from build123d import *

# Parameters (mm, degrees)
EXTRUDE_1_DEPTH     = 30
FILLET_1_R          = 1
SKETCH_3_R          = 1.6
CUT_EXTRUDE_1_DEPTH = 4


with BuildPart() as part:
    # 草图1 → 凸台-拉伸1 (new body)
    with BuildSketch(Plane.XY):
        Polygon((-34.18476969, 24.74285776), (-14.18476969, 24.74285776), (-14.18476969, 16.74285776), (-21.48476969, 16.74285776), (-19.68476969, 18.99285776), (-28.68476969, 18.99285776), (-26.88476969, 16.74285776), (-34.18476969, 16.74285776), align=None)
    extrude(amount=EXTRUDE_1_DEPTH)

    # 圆角1
    fillet_1_edges = [part.edges().sort_by_distance(p)[0] for p in [
        (-34.18476969, 24.74285776, 15),
        (-14.18476969, 24.74285776, 15),
        (-14.18476969, 16.74285776, 15),
        (-34.18476969, 16.74285776, 15),
    ]]
    fillet(fillet_1_edges, radius=FILLET_1_R)

    # 草图3 → 切除-拉伸1 (cut)
    with BuildSketch(Plane(origin=(0, 24.74285776, 0), x_dir=(1, 0, 0), z_dir=(0, 1, 0))):
        with Locations(Location((-31.68476969, -10, 0), (0, 0, 270))):
            Circle(SKETCH_3_R)
        with Locations(Location((-31.68476969, -20, 0), (0, 0, 270))):
            Circle(SKETCH_3_R)
        with Locations(Location((-16.68476969, -10, 0), (0, 0, 270))):
            Circle(SKETCH_3_R)
        with Locations(Location((-16.68476969, -20, 0), (0, 0, 270))):
            Circle(SKETCH_3_R)
        with Locations(Location((-24.18476969, -26, 0), (0, 0, 270))):
            Circle(SKETCH_3_R)
    extrude(amount=-CUT_EXTRUDE_1_DEPTH, mode=Mode.SUBTRACT)


solid = part.part
Work out the finished part from the listing and answer in its coordinate system (mm). A direction names the side the tool comes from. Round coordinates to 2 decimals unless told otherwise and drop trailing zeros. Write each loop counter-clockwise with the first axis right and the second up, starting at its lowest first coordinate (ties: lowest second). Pieces come first, ordered by that corner, then holes. Notation, with made-up numbers: (89, 4) -> (135, 4) arc R19 ccw to (135, 35) -> close; hole circle Ø1 at (61, 10). An arc over 180 degrees is marked (long way). Answer as CSV lines item,"result". Start each with the question number.
(1) The part is cut by section C-C, the plane z = 5. Give the vertices of the cut face in (x, y), then the cut area to 3 significant figures.
(2) The part is cut by section B-B, the plane x = -23. Give the vertices of the cut face in (y, z), then the cut area to 3 significant figures.
(3) Find the intervals of material crossed by probe 1 along Z at (x, y) = (-15.25, 21.5); probe 2 along Y at (x, z) = (-24.25, 6.5); probe 3 along Z at (x, y) = (-25.25, 23.25), in increasing order.
(4) A tool of negligible diameter and unlimited length cuts with its end or side. For faces 4 (the flat face through (-27.797, 17.884, 14.79)), 5 (the flat face through (-18, 16.743, 15)), 6 (the flat face through (-17, 20.743, 20)), from which of +Z, -Z, +X, -X, +Y, -Y can it reach the whole face along a straight path? Write none if from no direction.
(5) The mould has two halves that part along X. Classify faces 1 (the flat face through (-24, 18.993, 15)), 2 (the flat face through (-30, 16.743, 15)), 3 (the flat face through (-14.185, 21, 15)): +X half, -X half, draft (parallel to the pull), parting line (faces both ways), or undercut.
(6) The part is cut by section D-D, the plane z = 20. Give the vertices of the cut face in (x, y).
(7) Each of these flat-tipped pins is pushed along its axis until it touches: pin 1 (2.5 mm diameter, centred on x = -26.5, z = 11.5, fed in from -Y); pin 2 (1 mm diameter, centred on x = -16.5, z = 10.5, fed in from +Y). Where does it stop, or does it pass through?
(8) The part is cut by section A-A, the plane z = 26. Give the vertices of the cut face in (x, y), then the cut area to 3 significant figures.
Output values:
1,outline,"(-34.18, 17.74) arc R1 ccw to (-33.18, 16.74) -> (-26.88, 16.74) -> (-28.68, 18.99) -> (-19.68, 18.99) -> (-21.48, 16.74) -> (-15.18, 16.74) arc R1 ccw to (-14.18, 17.74) -> (-14.18, 23.74) arc R1 ccw to (-15.18, 24.74) -> (-33.18, 24.74) arc R1 ccw to (-34.18, 23.74) -> close"
1,area,"143 mm²"
2,outline,"(18.99, 0) -> (24.74, 0) -> (24.74, 24.92) -> (20.74, 24.92) -> (20.74, 27.08) -> (24.74, 27.08) -> (24.74, 30) -> (18.99, 30) -> close"
2,area,"164 mm²"
3,probe 1,"z = 0 to 9.29, 10.71 to 19.29, 20.71 to 30"
3,probe 2,"y = 18.99 to 24.74"
3,probe 3,"z = 0 to 24.81, 27.19 to 30"
4,face 4,"+Z, -Z"
4,face 5,"+Z, -Z, +X, -X, -Y"
4,face 6,"+Y"
5,face 1,"undercut"
5,face 2,"draft"
5,face 3,"+X half"
6,outline,"(-34.18, 17.74) arc R1 ccw to (-33.18, 16.74) -> (-26.88, 16.74) -> (-28.68, 18.99) -> (-19.68, 18.99) -> (-21.48, 16.74) -> (-15.18, 16.74) arc R1 ccw to (-14.18, 17.74) -> (-14.18, 23.74) arc R1 ccw to (-15.08, 24.74) -> (-15.08, 20.74) -> (-18.28, 20.74) -> (-18.28, 24.74) -> (-30.08, 24.74) -> (-30.08, 20.74) -> (-33.28, 20.74) -> (-33.28, 24.74) arc R1 ccw to (-34.18, 23.74) -> close"
7,pin 1,"stops at y = 16.74"
7,pin 2,"stops at y = 20.74"
8,outline,"(-34.18, 17.74) arc R1 ccw to (-33.18, 16.74) -> (-26.88, 16.74) -> (-28.68, 18.99) -> (-19.68, 18.99) -> (-21.48, 16.74) -> (-15.18, 16.74) arc R1 ccw to (-14.18, 17.74) -> (-14.18, 23.74) arc R1 ccw to (-15.18, 24.74) -> (-22.58, 24.74) -> (-22.58, 20.74) -> (-25.78, 20.74) -> (-25.78, 24.74) -> (-33.18, 24.74) arc R1 ccw to (-34.18, 23.74) -> close"
8,area,"130 mm²"
